```python
from build123d import *

# Parameters (mm, degrees)
F0_W           = 6.798369
F0_H           = 6.798369
F0_W_2         = 7.405656
F0_H_2         = 7.405656
F0_W_3         = 7.433599
F0_H_3         = 7.433599
F0_W_4         = 7.622234
F0_H_4         = 7.622235
F0_W_5         = 7.339932
F0_H_5         = 7.339932
F2_SIZE        = 5.08
F3_SIZE        = 5.08
F4_R           = 5.08
F7_D           = 6.35
F7_CSINK_D     = 12.7
F7_CSINK_ANGLE = 90
F8_R           = 5.08


with BuildPart() as f1:
    # F0 (on Front) → F1 (revolve)
    with BuildSketch(Plane.XZ):
        Polygon((-65.516091, 0), (-51.718292, 0), (-51.718292, 51.718292), (-32.323933, 51.718292), (-32.323933, 77.577439), (-44.875035, 77.577439), (-44.875035, 91.161532), (0, 91.161532), (0, 131.179577), (0, 143.122849), (-150.327997, 143.122849), (-150.327997, 131.179577), (-104.88727, 131.179577), (-104.88727, 0), align=None)
        with Locations((-70.299634, 10.931312)):
            Rectangle(F0_W, F0_H, mode=Mode.SUBTRACT)
        with Locations((-70.299634, 24.901313)):
            Rectangle(F0_W_2, F0_H_2, mode=Mode.SUBTRACT)
        with Locations((-70.299634, 38.871313)):
            Rectangle(F0_W_2, F0_H_2, mode=Mode.SUBTRACT)
        with Locations((-60.103797, 51.828418)):
            Rectangle(F0_W_3, F0_H_3, mode=Mode.SUBTRACT)
        with Locations((-40.06014, 64.785522)):
            Rectangle(F0_W_4, F0_H_4, mode=Mode.SUBTRACT)
        with Locations((-54.457691, 77.742626)):
            Rectangle(F0_W_5, F0_H_5, mode=Mode.SUBTRACT)
        with Locations((-54.457691, 90.69973)):
            Rectangle(F0_W_5, F0_H_5, mode=Mode.SUBTRACT)
    revolve(axis=Axis((0, 0, 81.092189), (0, 0, 1)))

    # F2
    f2_edges = [f1.edges().sort_by_distance(p)[0] for p in [
        (51.718292, 0, 0),
    ]]
    chamfer(f2_edges, length=F2_SIZE)

    # F3
    f3_edges = [f1.edges().sort_by_distance(p)[0] for p in [
        (32.323933, 0, 51.718292),
        (32.323933, 0, 77.577439),
    ]]
    chamfer(f3_edges, length=F3_SIZE)

    # F4
    f4_edges = [f1.edges().sort_by_distance(p)[0] for p in [
        (51.718292, 0, 51.718292),
    ]]
    fillet(f4_edges, radius=F4_R)

    # F7 (through all)
    with Locations(Plane(origin=(0, 0, 131.179577), x_dir=(1, 0, 0), z_dir=(0, 0, -1))):
        with Locations((-98.854152, 98.957022), (99.06, 98.957022), (99.06, -99.163085), (-99.06, -98.957022)):
            CounterSinkHole(F7_D / 2, F7_CSINK_D / 2, counter_sink_angle=F7_CSINK_ANGLE)

    # F8
    f8_edges = [f1.edges().sort_by_distance(p)[0] for p in [
        (104.88727, 0, 131.179577),
    ]]
    fillet(f8_edges, radius=F8_R)


solid = f1.part
```
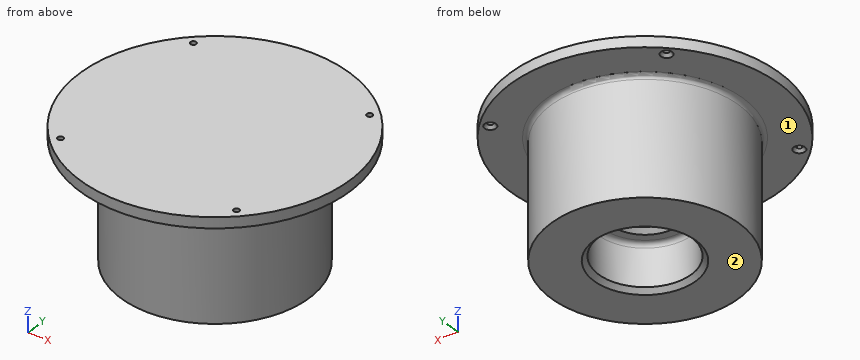
Design review of the part built by this model. Coordinates are the model's own, in mm. Face numbers are marked on the shaded views. A direction names the side the tool comes from. Round coordinates to 2 decimals unless told otherwise and drop trailing zeros. Order: outer loops, then holes, each group sorted by start corner. A loop starts at its lowest first (then second) coordinate and runs counter-clockwise, first axis right, second up. Notation, with made-up numbers: (48.5, 51) - (64.5, 51) arc R19 ccw to (64.5, 67) - close; hole circle Ø7 at (10.25, 57). An arc over 180 degrees is marked (long way). Return JSON: item names as keys, results as strings.
Q1. Consider section D-D on x = 118.5. Write out the cut boundary in (y, z).
Computed values:
{"outline": "(-92.5, 131.18) - (92.5, 131.18) - (92.5, 143.12) - (-92.5, 143.12) - close"}
Q2. Consider section C-C on z = 107.5. Write out the cut boundary in (x, y).
Computed values:
{"outline": "circle Ø209.77 at (0, 0)"}
Q3. For pin 1 Ø5 at (x, y) = (116.5, -21) entering from -Z; pin 2 Ø1 at (x, z) = (-37, 117) entering from +Y; pin 3 Ø4 at (y, z) = (-12.5, 111) entering from +X; pin 4 Ø2 at (x, y) = (-61.5, -27) entering from -Z, all flat-tipped, find the tip position at first contact; note any pin that passes through.
Computed values:
{"pin 1": "stops at z = 131.18", "pin 2": "stops at y = 98.33", "pin 3": "stops at x = 104.36", "pin 4": "stops at z = 0"}
Q4. Consider section A-A on y = 0. Give the number of separate pieces and of enclosed holes in the cut face, plus the area to 3 significant figures.
Computed values:
{"separate pieces": "1", "enclosed holes": "14", "area": "22,100 mm2"}
Q5. Machinability: for the marked faces 1 and 2, which of the approach directions +Z, -Z, +X, -X, +Y, -Y give a long, thin tool a straight path to every point of the face, cutting with its end or side? Answer none if there is none.
Computed values:
{"face 1": "-Z", "face 2": "-Z, +X, -X, +Y, -Y"}
Q6. Wall thickness on L1, parallel to X at y = 0, z = 62; L2, parallel to Z at x = -52, y = 45; L3, parallel to Y at x = 0, z = 10: over which ranges is each line inside the solid? List them lowest first. Write a range as [from, to].
Computed values:
{"L1": "x = [-104.89, -43.87], [-36.25, -32.32], [32.32, 36.25], [43.87, 104.89]", "L2": "z = [0, 7.53], [14.33, 21.2], [28.6, 35.17], [42.57, 143.12]", "L3": "y = [-104.89, -73.7], [-66.9, -51.72], [51.72, 66.9], [73.7, 104.89]"}
